Here's how the part is built. I have some questions about the finished solid (model axes, mm). A direction names the side the tool comes from. Round coordinates to 2 decimals unless told otherwise and drop trailing zeros. Loops run counter-clockwise (first coordinate to the right, second up) from the corner with the lowest first, then second, coordinate; pieces in that order, holes last. Notation, with made-up numbers: (72.25, -17.5) -> (97.25, -17.5) arc R32 cw to (97.25, 21.5) -> close; hole circle Ø11 at (-29.75, 9). An arc over 180 degrees is marked (long way). Use one line per item in the form item = value. Start each with the question number.
Item 1: If we section it at B-B (x = 16.5): Write out the boundary of the cut face in (y, z), then the cut area to 3 significant figures.
Item 2: If I drill on L1, parallel to Z at x = 64.77, y = 13 (1 decimal); L2, parallel to Z at x = 58.5, y = 14.25; L3, parallel to X at y = 4, z = -38, over which ranges is the centre line in solid material (lowest first)? Write a range as [from, to].
Item 3: I'm going to push flat-ended pins straight in: pin 1 Ø0.6 at (x, z) = (29, -23.5) entering from +Y; pin 2 Ø1 at (x, z) = (5, -41) entering from +Y; pin 3 Ø2 at (x, z) = (57.5, -32.5) entering from +Y; pin 4 Ø3 at (x, z) = (64.77, -40.64) entering from +Y. Where does each tip first touch, or does it pass through?
Item 4: If we section it at A-A (y = 14): State how many separate pieces and enclosed holes the cut face has, then the cut area to 3 significant figures.
Item 5: For faces 1 (the face through (34, 9, 0)), 2 (the face through (63.84, 13.89, -5.29)), 3 (the face through (1, 16, -11.748)), which set-ups out of +Z, -Z, +X, -X, +Y, -Y let a thin tool reach every point of the face, with its end or its side?
Item 6: If we section it at C-C (z = -19.5): Write out the boundary of the cut face in (x, y).
Item 7: Thinking about a two-plate mould opening in X: for faces 4 (the face through (54, 2.794, -13)), 5 (the face through (35, 17.018, -45)), which applies, released by +X, released by -X, zero draft, split by the parting line, or undercut?
```python
from build123d import *

# Parameters (mm, degrees)
SKETCH2_W            = 69.85
SKETCH2_H            = 45.72
BOSS_EXTRUDE1_DEPTH  = 17.018
SKETCH3_W            = 64.77
SKETCH3_H            = 40.64
CUT_EXTRUDE1_DEPTH   = 14.224
SKETCH13_R           = 1.905
BOSS_EXTRUDE5_DEPTH  = 6.35
SKETCH14_R           = 0.9525
CUT_EXTRUDE4_DEPTH   = 6.35
CUT_EXTRUDE5_DEPTH   = 2.54
FILLET1_R            = 1.27
SKETCH18_R           = 1.905
BOSS_EXTRUDE11_DEPTH = 14.224
SKETCH19_R           = 0.9525
CUT_EXTRUDE6_DEPTH   = 6.35


with BuildPart() as part:
    # Sketch2 → Boss-Extrude1 (new body)
    with BuildSketch(Plane(origin=(0, 0, 0), x_dir=(1, 0, 0), z_dir=(0, 1, 0))):
        with Locations((34.925, 22.86)):
            Rectangle(SKETCH2_W, SKETCH2_H)
    extrude(amount=BOSS_EXTRUDE1_DEPTH)

    # Sketch3 → Cut-Extrude1 (cut)
    with BuildSketch(Plane(origin=(0, 17.018, 0), x_dir=(1, 0, 0), z_dir=(0, 1, 0))):
        with Locations((34.925, 22.86)):
            Rectangle(SKETCH3_W, SKETCH3_H)
    extrude(amount=-CUT_EXTRUDE1_DEPTH, mode=Mode.SUBTRACT)

    # Sketch13 → Boss-Extrude5 (add)
    with BuildSketch(Plane(origin=(0, 2.794, 0), x_dir=(1, 0, 0), z_dir=(0, 1, 0))):
        with Locations(Location((57.277, 32.3596, 0), (0, 0, 270))):
            Circle(SKETCH13_R)
        with Locations(Location((53.7972, 12.8778, 0), (0, 0, 270))):
            Circle(SKETCH13_R)
        with Locations(Location((28.7782, 23.876, 0), (0, 0, 270))):
            Circle(SKETCH13_R)
    extrude(amount=BOSS_EXTRUDE5_DEPTH)

    # Sketch14 → Cut-Extrude4 (cut)
    with BuildSketch(Plane(origin=(0, 9.144, 0), x_dir=(1, 0, 0), z_dir=(0, 1, 0))):
        with Locations(Location((57.277, 32.3596, 0), (0, 0, 270))):
            Circle(SKETCH14_R)
        with Locations(Location((53.7972, 12.8778, 0), (0, 0, 270))):
            Circle(SKETCH14_R)
        with Locations(Location((28.7782, 23.876, 0), (0, 0, 270))):
            Circle(SKETCH14_R)
    extrude(amount=-CUT_EXTRUDE4_DEPTH, mode=Mode.SUBTRACT)

    # Sketch17 → Cut-Extrude5 (cut)
    with BuildSketch(Plane.ZY):
        with BuildLine():
            Line((-16.1925, 14.7955), (-16.1925, 17.018))
            Line((-16.1925, 17.018), (-11.7475, 17.018))
            Line((-11.7475, 17.018), (-11.7475, 14.7955))
            ThreePointArc((-11.7475, 14.7955), (-13.97, 12.573), (-16.1925, 14.7955))
        make_face()
    extrude(amount=-CUT_EXTRUDE5_DEPTH, mode=Mode.SUBTRACT)

    # Fillet1
    fillet1_edges = [part.edges().sort_by_distance(p)[0] for p in [
        (34.925, 0, -45.72),
        (69.85, 0, -22.86),
        (34.925, 0, 0),
        (0, 0, -22.86),
        (0, 8.509, -45.72),
        (69.85, 8.509, -45.72),
        (69.85, 8.509, 0),
        (0, 8.509, 0),
    ]]
    fillet(fillet1_edges, radius=FILLET1_R)

    # Sketch18 → Boss-Extrude11 (add)
    with BuildSketch(Plane(origin=(0, 2.794, 0), x_dir=(1, 0, 0), z_dir=(0, 1, 0))):
        with Locations(Location((5.08, 40.64, 0), (0, 0, 90))):
            Circle(SKETCH18_R)
        with Locations(Location((64.77, 40.64, 0), (0, 0, 90))):
            Circle(SKETCH18_R)
        with Locations(Location((5.08, 5.08, 0), (0, 0, 90))):
            Circle(SKETCH18_R)
        with Locations(Location((64.77, 5.08, 0), (0, 0, 90))):
            Circle(SKETCH18_R)
    extrude(amount=BOSS_EXTRUDE11_DEPTH)

    # Sketch19 → Cut-Extrude6 (cut)
    with BuildSketch(Plane(origin=(0, 17.018, 0), x_dir=(1, 0, 0), z_dir=(0, 1, 0))):
        with Locations(Location((5.08, 40.64, 0), (0, 0, 270))):
            Circle(SKETCH19_R)
        with Locations(Location((64.77, 40.64, 0), (0, 0, 270))):
            Circle(SKETCH19_R)
        with Locations(Location((64.77, 5.08, 0), (0, 0, 270))):
            Circle(SKETCH19_R)
        with Locations(Location((5.08, 5.08, 0), (0, 0, 270))):
            Circle(SKETCH19_R)
    extrude(amount=-CUT_EXTRUDE6_DEPTH, mode=Mode.SUBTRACT)


solid = part.part
```
Values found:
q1.outline = (0, -44.45) arc R1.27 ccw to (1.27, -45.72) -> (17.02, -45.72) -> (17.02, -43.18) -> (2.79, -43.18) -> (2.79, -2.54) -> (17.02, -2.54) -> (17.02, 0) -> (1.27, 0) arc R1.27 ccw to (0, -1.27) -> close
q1.area = 199 mm2
q2.L1 = [-45.7, -43.2], [-42.5, -41.6], [-39.7, -38.7], [-7, -6], [-4.1, -3.2], [-2.5, 0]
q2.L2 = [-45.72, -43.18], [-2.54, 0]
q2.L3 = [0, 2.54], [67.31, 69.85]
q3.pin_1 = 2.79
q3.pin_2 = 10.67
q3.pin_3 = 9.14
q3.pin_4 = 17.02
q4.separate_pieces = 5
q4.enclosed_holes = 4
q4.area = 584 mm2
q5.face_1 = +Z, +X, -X, +Y, -Y
q5.face_2 = +Y
q5.face_3 = -X, +Y
q6.outline = (0, 1.27) arc R1.27 ccw to (1.27, 0) -> (68.58, 0) arc R1.27 ccw to (69.85, 1.27) -> (69.85, 17.02) -> (67.31, 17.02) -> (67.31, 2.79) -> (2.54, 2.79) -> (2.54, 17.02) -> (0, 17.02) -> close
q7.face_4 = undercut
q7.face_5 = zero draft
